Check sheet for the modelled part. Datum: model origin and axes. Units: mm. Face numbers are marked on the shaded views. A direction names the side the tool comes from. Give positions to 0.01 mm unless a question says otherwise; leave off trailing zeros. Order: outer loops, then holes, each group sorted by start corner. A loop starts at its lowest first (then second) coordinate and runs counter-clockwise, first axis right, second up.
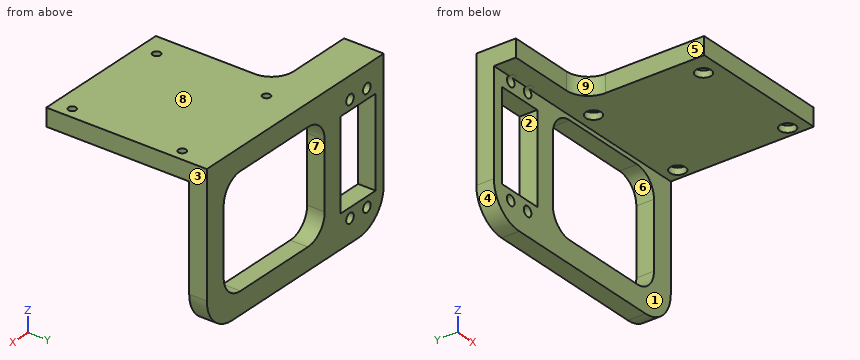
from build123d import *

# Parameters (mm, degrees)
SKETCH2_W           = 105
SKETCH2_H           = 70
BOSS_EXTRUDE1_DEPTH = 8
SKETCH4_W           = 105
SKETCH4_H           = 8
BOSS_EXTRUDE2_DEPTH = 65
SKETCH6_R           = 1.75
CUT_EXTRUDE1_DEPTH  = 10
SKETCH7_R           = 3.5
CUT_EXTRUDE2_DEPTH  = 3
SKETCH9_W           = 21
SKETCH9_H           = 40.5
CUT_EXTRUDE3_DEPTH  = 10
SKETCH10_R          = 2.25
CUT_EXTRUDE4_DEPTH  = 10
FILLET1_R           = 15
FILLET2_R           = 15
SKETCH12_W          = 60
SKETCH12_H          = 50
CUT_EXTRUDE5_DEPTH  = 10
FILLET3_R           = 10
FILLET4_R           = 10
FILLET5_R           = 10
FILLET6_R           = 10
SKETCH13_W          = 40
SKETCH13_H          = 55
CUT_EXTRUDE6_DEPTH  = 10
FILLET7_R           = 10


with BuildPart() as part:
    # Sketch2 → Boss-Extrude1 (new body)
    with BuildSketch(Plane(origin=(0, 0, 0), x_dir=(1, 0, 0), z_dir=(0, 1, 0))):
        with Locations((37.5, 2.5)):
            Rectangle(SKETCH2_W, SKETCH2_H)
    extrude(amount=BOSS_EXTRUDE1_DEPTH)

    # Sketch4 → Boss-Extrude2 (add)
    with BuildSketch(Plane(origin=(0, 0, 0), x_dir=(-1, 0, 0), z_dir=(0, -1, 0))):
        with Locations((-37.5, -28.5)):
            Rectangle(SKETCH4_W, SKETCH4_H)
    extrude(amount=BOSS_EXTRUDE2_DEPTH)

    # Sketch6 → Cut-Extrude1 (cut)
    with BuildSketch(Plane(origin=(0, 0, 24.5), x_dir=(-1, 0, 0), z_dir=(0, 0, -1))):
        with Locations((-85, -7)):
            Circle(SKETCH6_R)
        with Locations((-35, -7)):
            Circle(SKETCH6_R)
        with Locations((-85, -57)):
            Circle(SKETCH6_R)
        with Locations((-35, -57)):
            Circle(SKETCH6_R)
    extrude(amount=-CUT_EXTRUDE1_DEPTH, mode=Mode.SUBTRACT)

    # Sketch7 → Cut-Extrude2 (cut)
    with BuildSketch(Plane(origin=(0, 0, 24.5), x_dir=(-1, 0, 0), z_dir=(0, 0, -1))):
        with Locations((-85, -7)):
            Circle(SKETCH7_R)
        with Locations((-35, -7)):
            Circle(SKETCH7_R)
        with Locations((-35, -57)):
            Circle(SKETCH7_R)
        with Locations((-85, -57)):
            Circle(SKETCH7_R)
    extrude(amount=-CUT_EXTRUDE2_DEPTH, mode=Mode.SUBTRACT)

    # Sketch9 → Cut-Extrude3 (cut)
    with BuildSketch(Plane(origin=(0, 8, 0), x_dir=(1, 0, 0), z_dir=(0, 1, 0))):
        with Locations((0.25, 2.25)):
            Rectangle(SKETCH9_W, SKETCH9_H)
    extrude(amount=-CUT_EXTRUDE3_DEPTH, mode=Mode.SUBTRACT)

    # Sketch10 → Cut-Extrude4 (cut)
    with BuildSketch(Plane(origin=(0, 8, 0), x_dir=(1, 0, 0), z_dir=(0, 1, 0))):
        with Locations(Location((-5, 27, 0), (0, 0, 270))):
            Circle(SKETCH10_R)
        with Locations(Location((5, 27, 0), (0, 0, 270))):
            Circle(SKETCH10_R)
        with Locations(Location((-5, -22.5, 0), (0, 0, 270))):
            Circle(SKETCH10_R)
        with Locations(Location((5, -22.5, 0), (0, 0, 270))):
            Circle(SKETCH10_R)
    extrude(amount=-CUT_EXTRUDE4_DEPTH, mode=Mode.SUBTRACT)

    # Fillet1
    fillet1_edges = [part.edges().sort_by_distance(p)[0] for p in [
        (90, 4, -37.5),
    ]]
    fillet(fillet1_edges, radius=FILLET1_R)

    # Fillet2
    fillet2_edges = [part.edges().sort_by_distance(p)[0] for p in [
        (-15, 4, -37.5),
    ]]
    fillet(fillet2_edges, radius=FILLET2_R)

    # Sketch12 → Cut-Extrude5 (cut)
    with BuildSketch(Plane(origin=(0, 8, 0), x_dir=(1, 0, 0), z_dir=(0, 1, 0))):
        with Locations((50, 2.5)):
            Rectangle(SKETCH12_W, SKETCH12_H)
    extrude(amount=-CUT_EXTRUDE5_DEPTH, mode=Mode.SUBTRACT)

    # Fillet3
    fillet3_edges = [part.edges().sort_by_distance(p)[0] for p in [
        (20, 4, 22.5),
    ]]
    fillet(fillet3_edges, radius=FILLET3_R)

    # Fillet4
    fillet4_edges = [part.edges().sort_by_distance(p)[0] for p in [
        (80, 4, 22.5),
    ]]
    fillet(fillet4_edges, radius=FILLET4_R)

    # Fillet5
    fillet5_edges = [part.edges().sort_by_distance(p)[0] for p in [
        (80, 4, -27.5),
    ]]
    fillet(fillet5_edges, radius=FILLET5_R)

    # Fillet6
    fillet6_edges = [part.edges().sort_by_distance(p)[0] for p in [
        (20, 4, -27.5),
    ]]
    fillet(fillet6_edges, radius=FILLET6_R)

    # Sketch13 → Cut-Extrude6 (cut)
    with BuildSketch(Plane(origin=(0, 0, 24.5), x_dir=(-1, 0, 0), z_dir=(0, 0, -1))):
        with Locations((-5, -37.5)):
            Rectangle(SKETCH13_W, SKETCH13_H)
    extrude(amount=-CUT_EXTRUDE6_DEPTH, mode=Mode.SUBTRACT)

    # Fillet7
    fillet7_edges = [part.edges().sort_by_distance(p)[0] for p in [
        (25, -10, 28.5),
    ]]
    fillet(fillet7_edges, radius=FILLET7_R)


solid = part.part
1) Section check D-D, the plane y = -16.5. Record the cut outline in (x, z), then the cut area to 3 significant figures.
Recorded:
outline: (24.37, 24.5) - (90, 24.5) - (90, 32.5) - (24.37, 32.5) - close
area: 525 mm2
2) Section check C-C, the plane x = 42. Record the cut outline in (y, z), then the cut area to 3 significant figures.
Recorded:
outline: (-65, 24.5) - (0, 24.5) - (0, 22.5) - (8, 22.5) - (8, 32.5) - (-65, 32.5) - close; (0, -37.5) - (8, -37.5) - (8, -27.5) - (0, -27.5) - close
area: 680 mm2
3) Material ranges on L1, parallel to Y at x = 85, z = 28.8; L2, parallel to Y at x = 85, z = 25; L3, parallel to X at y = 5, z = -19, recorded low to high.
Recorded:
L1: y = -65 to -58.75, -55.25 to -8.75, -5.25 to 8
L2: y = -65 to -60.5, -53.5 to -10.5, -3.5 to 8
L3: x = -15 to -10.25, 10.75 to 20.11, 79.89 to 90
4) Set-up check for the marked faces 1, 2, 3, 4 and 5: record each of +Z, -Z, +X, -X, +Y, -Y from which the full face is reachable in a straight line by a thin tool's end or side.
Recorded:
face 1: -Z, +X, -X, -Y
face 2: +Y, -Y
face 3: +Z, -Z, +X, +Y, -Y
face 4: -Z, -X, +Y, -Y
face 5: +Z, -Z, -X, -Y
5) Section check B-B, the plane z = 11. Record the cut outline in (x, y), then the cut area to 3 significant figures.
Recorded:
outline: (-15, 0) - (-10.25, 0) - (-10.25, 8) - (-15, 8) - close; (10.75, 0) - (20, 0) - (20, 8) - (10.75, 8) - close; (80, 0) - (90, 0) - (90, 8) - (80, 8) - close
area: 192 mm2
6) Draft check along Z on the marked faces 6, 7, 8 and 9. Enter one of: +Z half, -Z half, draft (parallel to the pull), parting line (faces both ways), or undercut.
Recorded:
face 6: undercut
face 7: undercut
face 8: +Z half
face 9: draft
7) Section check A-A, the plane y = -7. Record the cut outline in (x, z).
Recorded:
outline: (-15, 24.5) - (31.5, 24.5) - (31.5, 27.5) - (33.25, 27.5) - (33.25, 32.5) - (-15, 32.5) - close; (36.75, 27.5) - (38.5, 27.5) - (38.5, 24.5) - (81.5, 24.5) - (81.5, 27.5) - (83.25, 27.5) - (83.25, 32.5) - (36.75, 32.5) - close; (86.75, 27.5) - (88.5, 27.5) - (88.5, 24.5) - (90, 24.5) - (90, 32.5) - (86.75, 32.5) - close
8) Depth check by flat-ended pin: pin 1 Ø5 at (x, y) = (40.5, -14.5) entering from -Z; pin 2 Ø5 at (x, z) = (79, -17.5) entering from -Y; pin 3 Ø9 at (y, z) = (-31.5, 28) entering from -X; pin 4 Ø6 at (y, z) = (-1, -6.5) entering from +X. Enter the tip coordinate at first touch or a pass-through.
Recorded:
pin 1: stops at z = 24.5
pin 2: stops at y = 0
pin 3: stops at x = 25
pin 4: stops at x = 90
